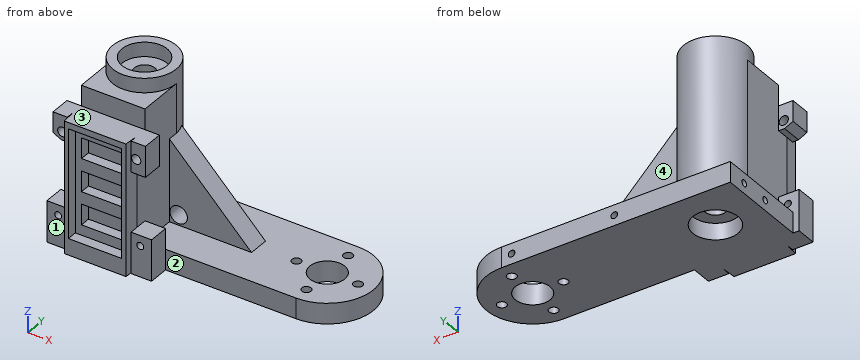
```python
from build123d import *

# Parameters (mm, degrees)
SKETCH1_W                = 26
SKETCH1_H                = 53
SKETCH1_W_2              = 20
SKETCH1_H_2              = 10
BOSS_EXTRUDE1_DEPTH      = 5
SKETCH2_W                = 31
SKETCH2_H                = 59
SKETCH2_W_2              = 26
SKETCH2_H_2              = 53
BOSS_EXTRUDE2_DEPTH      = 10
SKETCH3_W                = 31
SKETCH3_H                = 59
BOSS_EXTRUDE3_DEPTH      = 3
CHAMFER1_SIZE            = 0.5
CHAMFER1_SIZE2           = 7.150333128
SKETCH10_W               = 7
SKETCH10_H               = 15
SKETCH10_R               = 2.25
BOSS_EXTRUDE7_DEPTH      = 10
SKETCH11_W               = 7
SKETCH11_H               = 3
CUT_EXTRUDE4_DEPTH       = 10
CHAMFER2_SIZE            = 2
CHAMFER2_SIZE2           = 4.100607683
BOSS_EXTRUDE8_REACH      = 69.567
SKETCH12_W               = 10
SKETCH12_H               = 15
SKETCH12_R               = 1.676379865
BOSS_EXTRUDE9_START      = -56
SKETCH15_R               = 8.5
SKETCH15_R_2             = 2.25
SKETCH15_R_3             = 11
BOSS_EXTRUDE9_DEPTH      = 5
BOSS_EXTRUDE9_DEPTH_BACK = 5
SKETCH16_R               = 2.25
SKETCH16_R_2             = 8.5
SKETCH16_R_3             = 5
BOSS_EXTRUDE10_DEPTH     = 2
SKETCH17_R               = 5
BOSS_EXTRUDE11_DEPTH     = 64
RIB2_REACH               = 123.175
SKETCH20_WALL_W          = 300.919527638
SKETCH20_WALL_H          = 10
BOSS_EXTRUDE12_DEPTH     = 5
SKETCH22_R               = 15.5
SKETCH22_R_2             = 11
BOSS_EXTRUDE13_DEPTH     = 7
SKETCH23_R               = 4.25
CUT_EXTRUDE5_DEPTH       = 29
SKETCH24_R               = 1.6
CUT_EXTRUDE6_DEPTH       = 8
SKETCH25_R               = 1.6
CUT_EXTRUDE7_DEPTH       = 8


with BuildPart() as part:
    # Sketch1 → Boss-Extrude1 (new body)
    with BuildSketch(Plane(origin=(0, 0, 0), x_dir=(1, 0, 0), z_dir=(0, 1, 0))):
        with Locations((-13, 26.5)):
            Rectangle(SKETCH1_W, SKETCH1_H)
        with Locations((-13, 27)):
            Rectangle(SKETCH1_W_2, SKETCH1_H_2, mode=Mode.SUBTRACT)
        with Locations((-13, 43)):
            Rectangle(SKETCH1_W_2, SKETCH1_H_2, mode=Mode.SUBTRACT)
        with Locations((-13, 11)):
            Rectangle(SKETCH1_W_2, SKETCH1_H_2, mode=Mode.SUBTRACT)
    extrude(amount=BOSS_EXTRUDE1_DEPTH)

    # Sketch2 → Boss-Extrude2 (add)
    with BuildSketch(Plane(origin=(0, 5, 0), x_dir=(1, 0, 0), z_dir=(0, 1, 0))):
        with Locations((-13, 26.5)):
            Rectangle(SKETCH2_W, SKETCH2_H)
        with Locations((-13, 26.5)):
            Rectangle(SKETCH2_W_2, SKETCH2_H_2, mode=Mode.SUBTRACT)
    extrude(amount=-BOSS_EXTRUDE2_DEPTH)

    # Sketch3 → Boss-Extrude3 (add)
    with BuildSketch(Plane(origin=(0, 5, 0), x_dir=(1, 0, 0), z_dir=(0, 1, 0))):
        with Locations((-13, 26.5)):
            Rectangle(SKETCH3_W, SKETCH3_H)
    extrude(amount=BOSS_EXTRUDE3_DEPTH)

    # Chamfer1
    chamfer1_edges = [part.edges().sort_by_distance(p)[0] for p in [
        (-28.5, -5, -26.5),
        (2.5, -5, -26.5),
    ]]
    chamfer1_side = [part.faces().sort_by_distance(p)[0] for p in [
        (-13, -5, -55.333516692),
    ]]
    chamfer(chamfer1_edges, length=CHAMFER1_SIZE, length2=CHAMFER1_SIZE2, reference=chamfer1_side[0])

    # Sketch10 → Boss-Extrude7 (add)
    with BuildSketch(Plane(origin=(0, 8, 0), x_dir=(1, 0, 0), z_dir=(0, 1, 0))):
        with Locations((6, 4.5)):
            Rectangle(SKETCH10_W, SKETCH10_H)
        with Locations(Location((5, 5, 0), (0, 0, 270))):
            Circle(SKETCH10_R, mode=Mode.SUBTRACT)
        with Locations((-32, 4.5)):
            Rectangle(SKETCH10_W, SKETCH10_H)
        with Locations(Location((-31, 5, 0), (0, 0, 90))):
            Circle(SKETCH10_R, mode=Mode.SUBTRACT)
    extrude(amount=-BOSS_EXTRUDE7_DEPTH)

    # Sketch11 → Cut-Extrude4 (cut)
    with BuildSketch(Plane(origin=(0, 8, 0), x_dir=(1, 0, 0), z_dir=(0, 1, 0))):
        with Locations((-32, 10.5)):
            Rectangle(SKETCH11_W, SKETCH11_H)
    extrude(amount=-CUT_EXTRUDE4_DEPTH, mode=Mode.SUBTRACT)

    # Chamfer2
    chamfer2_edges = [part.edges().sort_by_distance(p)[0] for p in [
        (-35.5, 3, -9),
    ]]
    chamfer2_side = [part.faces().sort_by_distance(p)[0] for p in [
        (-35.5, 3, -3),
    ]]
    chamfer(chamfer2_edges, length=CHAMFER2_SIZE, length2=CHAMFER2_SIZE2, reference=chamfer2_side[0])

    # Boss-Extrude8: up to this face of the body (flat: up to its plane)
    boss_extrude8_end = Plane(part.part.faces().sort_by_distance((6, -2, 2.834470546))[0])
    # Sketch12 → Boss-Extrude8 (add, up to the picked face)
    with BuildSketch(Plane(origin=(0, 8, 0), x_dir=(1, 0, 0), z_dir=(0, 1, 0)), mode=Mode.PRIVATE) as boss_extrude8_sk1:
        with Locations((7.5, 48.5)):
            Rectangle(SKETCH12_W, SKETCH12_H)
        with Locations(Location((7, 46, 0), (0, 0, 270))):
            Circle(SKETCH12_R, mode=Mode.SUBTRACT)
    boss_extrude8_tool1 = split(extrude(boss_extrude8_sk1.sketch, amount=-BOSS_EXTRUDE8_REACH, mode=Mode.PRIVATE), bisect_by=boss_extrude8_end, keep=Keep.BOTH, mode=Mode.PRIVATE)
    # Sketch12 → Boss-Extrude8 (add, up to the picked face)
    with BuildSketch(Plane(origin=(0, 8, 0), x_dir=(1, 0, 0), z_dir=(0, 1, 0)), mode=Mode.PRIVATE) as boss_extrude8_sk2:
        with Locations((-33.5, 48.5)):
            Rectangle(SKETCH12_W, SKETCH12_H)
        with Locations(Location((-33, 46, 0), (0, 0, 270))):
            Circle(SKETCH12_R, mode=Mode.SUBTRACT)
    boss_extrude8_tool2 = split(extrude(boss_extrude8_sk2.sketch, amount=-BOSS_EXTRUDE8_REACH, mode=Mode.PRIVATE), bisect_by=boss_extrude8_end, keep=Keep.BOTH, mode=Mode.PRIVATE)
    add(boss_extrude8_tool1.solids().sort_by(Axis((7.531269, 8, -48.656347), (0, -1, 0)))[0])
    add(boss_extrude8_tool2.solids().sort_by(Axis((-33.531269, 8, -48.656347), (0, -1, 0)))[0])

    # Sketch15 → Boss-Extrude9 (add, two sides)
    with BuildSketch(Plane.XY.offset(BOSS_EXTRUDE9_START)) as boss_extrude9_sk:
        with BuildLine():
            Line((-13, 53), (76, 53))
            ThreePointArc((76, 53), (98.5, 30.5), (76, 8))
            Line((76, 8), (-13, 8))
            Line((-13, 8), (-35.5, 8))
            Line((-35.5, 8), (-35.5, 53))
            Line((-35.5, 53), (-13, 53))
        make_face()
        with Locations(Location((76, 30.5, 0), (0, 0, 180))):
            Circle(SKETCH15_R, mode=Mode.SUBTRACT)
        with Locations(Location((76, 45.5, 0), (0, 0, 180))):
            Circle(SKETCH15_R_2, mode=Mode.SUBTRACT)
        with Locations(Location((76, 15.5, 0), (0, 0, 180))):
            Circle(SKETCH15_R_2, mode=Mode.SUBTRACT)
        with Locations(Location((91, 30.5, 0), (0, 0, 180))):
            Circle(SKETCH15_R_2, mode=Mode.SUBTRACT)
        with Locations(Location((61, 30.5, 0), (0, 0, 180))):
            Circle(SKETCH15_R_2, mode=Mode.SUBTRACT)
        with Locations(Location((-13, 30.5, 0), (0, 0, 180))):
            Circle(SKETCH15_R_3, mode=Mode.SUBTRACT)
    extrude(amount=BOSS_EXTRUDE9_DEPTH)
    extrude(boss_extrude9_sk.sketch, amount=-BOSS_EXTRUDE9_DEPTH_BACK)

    # Sketch16 → Boss-Extrude10 (add)
    with BuildSketch(Plane.XY.offset(-51)):
        with BuildLine():
            Line((-35.5, 53), (-35.5, 8))
            Line((-35.5, 8), (12.5, 8))
            Line((12.5, 8), (76, 8))
            ThreePointArc((76, 8), (98.5, 30.5), (76, 53))
            Line((76, 53), (-35.5, 53))
        make_face()
        with Locations(Location((76, 45.5, 0), (0, 0, 180))):
            Circle(SKETCH16_R, mode=Mode.SUBTRACT)
        with Locations(Location((91, 30.5, 0), (0, 0, 180))):
            Circle(SKETCH16_R, mode=Mode.SUBTRACT)
        with Locations(Location((76, 15.5, 0), (0, 0, 180))):
            Circle(SKETCH16_R, mode=Mode.SUBTRACT)
        with Locations(Location((76, 30.5, 0), (0, 0, 180))):
            Circle(SKETCH16_R_2, mode=Mode.SUBTRACT)
        with Locations(Location((61, 30.5, 0), (0, 0, 180))):
            Circle(SKETCH16_R, mode=Mode.SUBTRACT)
        with Locations((-13, 30.5)):
            Circle(SKETCH16_R_3, mode=Mode.SUBTRACT)
    extrude(amount=-BOSS_EXTRUDE10_DEPTH)

    # Sketch17 → Boss-Extrude11 (add)
    with BuildSketch(Plane.XY.offset(-51)):
        with BuildLine():
            Line((-28.5, 30.5), (-28.5, 8))
            Line((-28.5, 8), (2.5, 8))
            Line((2.5, 8), (2.5, 30.5))
            ThreePointArc((2.5, 30.5), (-13, 46), (-28.5, 30.5))
        make_face()
        with Locations((-13, 30.5)):
            Circle(SKETCH17_R, mode=Mode.SUBTRACT)
    extrude(amount=BOSS_EXTRUDE11_DEPTH)

    # Sketch20 wall → Rib2 (add, up to next)
    with BuildSketch(Plane(origin=(22.5, 30.5, -31), x_dir=(-0.707106781187, 0, 0.707106781187), z_dir=(0.707106781187, 0, 0.707106781187)), mode=Mode.PRIVATE) as rib2_sk1:
        Rectangle(SKETCH20_WALL_W, SKETCH20_WALL_H)
    rib2_tool1 = extrude(rib2_sk1.sketch, amount=-RIB2_REACH, mode=Mode.PRIVATE) - part.part
    add(rib2_tool1.solids().sort_by_distance((22.5, 30.5, -31))[0])

    # Sketch21 → Boss-Extrude12 (add)
    with BuildSketch(Plane(origin=(0, 0, -56), x_dir=(-1, 0, 0), z_dir=(0, 0, -1))):
        Polygon((-2, -5), (28, -5), (28.5, 2.150333128), (28.5, -2), (38.5, -2), (38.5, 8), (35.5, 8), (-12.5, 8), (-12.5, -2), (-2.5, -2), (-2.5, 2.150333128), align=None)
    extrude(amount=BOSS_EXTRUDE12_DEPTH)

    # Sketch22 → Boss-Extrude13 (add)
    with BuildSketch(Plane.XY.offset(13)):
        with Locations((-13, 30.5)):
            Circle(SKETCH22_R)
        with Locations((-13, 30.5)):
            Circle(SKETCH22_R_2, mode=Mode.SUBTRACT)
    extrude(amount=BOSS_EXTRUDE13_DEPTH)

    # Sketch23 → Cut-Extrude5 (cut)
    with BuildSketch(Plane(origin=(0, 8, 0), x_dir=(1, 0, 0), z_dir=(0, 1, 0))):
        with Locations(Location((7, 46, 0), (0, 0, 270))):
            Circle(SKETCH23_R)
    extrude(amount=CUT_EXTRUDE5_DEPTH, mode=Mode.SUBTRACT)

    # Sketch24 → Cut-Extrude6 (cut)
    with BuildSketch(Plane.ZY.offset(35.5)):
        with Locations((-56, 28)):
            Circle(SKETCH24_R)
        with Locations((-56, 43)):
            Circle(SKETCH24_R)
    extrude(amount=-CUT_EXTRUDE6_DEPTH, mode=Mode.SUBTRACT)

    # Sketch25 → Cut-Extrude7 (cut)
    with BuildSketch(Plane(origin=(0, 53, 0), x_dir=(1, 0, 0), z_dir=(0, 1, 0))):
        with Locations(Location((71, 56, 0), (0, 0, 270))):
            Circle(SKETCH25_R)
        with Locations(Location((21, 56, 0), (0, 0, 270))):
            Circle(SKETCH25_R)
    extrude(amount=-CUT_EXTRUDE7_DEPTH, mode=Mode.SUBTRACT)


solid = part.part
```
Design review of the part built by this model. Coordinates are the model's own, in mm. Face numbers are marked on the shaded views. A direction names the side the tool comes from. Coordinates: 2 decimals unless noted, no trailing zeros. Order: outer loops, then holes, each group sorted by start corner. A loop starts at its lowest first (then second) coordinate and runs counter-clockwise, first axis right, second up. Notation, with made-up numbers: M 68,55.5 L 98,55.5 A18 ccw 98,85.5 Z; hole C 73.25,52.25 d10. An arc over 180 degrees is marked long. Answer as a JSON object with one key per item and string values. Group by question number.
1) Add section D-D, the plane z = 9.5. Write out the cut boundary in (x, y).
2) Add section B-B, the plane x = 91. Write out the cut boundary in (y, z).
3) Add section A-A, the plane z = -19. Write out the cut boundary in (x, y).
4) For pin 1 (5 mm diameter, centred on x = 33, z = -47.5, fed in from +Y); pin 2 (3 mm diameter, centred on x = -8.5, z = 7, fed in from -Y); pin 3 (1.5 mm diameter, centred on y = 8.5, z = -2, fed in from +X); pin 4 (2.5 mm diameter, centred on x = -33, z = -46, fed in from -Y), all flat-tipped, find the tip position at first contact; note any pin that passes through.
5) Add section C-C, the plane x = 21. Write out the cut boundary in (y, z), then the cut area to 3 significant figures.
6) Tool access review of the marked faces 1, 2, 3 and 4: name each direction out of +Z, -Z, +X, -X, +Y, -Y from which nothing blocks a thin tool from reaching the whole face with its end or side.
7) Wall thickness on L1, parallel to Y at x = 76, z = -55.25; L2, parallel to X at y = 2.75, z = -5; L3, parallel to Y at x = -33, z = -56: over which ranges is each line inside the solid? List them lowest first.
Computed values:
{
 "1": {"outline": "M -28.5,8 L 2.5,8 L 2.5,30.5 A15.5 ccw -28.5,30.5 Z; hole C -13,30.5 d10"},
 "2": {"outline": "M 13.73,-61 L 28.25,-61 L 28.25,-51 L 13.73,-51 Z; M 32.75,-61 L 47.27,-61 L 47.27,-51 L 32.75,-51 Z"},
 "3": {"outline": "M -28.5,2.15 L -28,-5 L -26,-5 L -26,0 L 0,0 L 0,-5 L 2,-5 L 2.5,2.15 L 2.5,25.5 L 10.5,25.5 L 10.5,35.5 L 1.67,35.5 A15.5 ccw -28.5,30.5 Z; hole C -13,30.5 d10"},
 "4": {"pin 1": "stops at y = 35.5", "pin 2": "stops at y = 8", "pin 3": "stops at x = 9.5", "pin 4": "passes through"},
 "5": {"outline": "M 8,-61 L 53,-61 L 53,-57.6 L 45,-57.6 L 45,-54.4 L 53,-54.4 L 53,-51 L 35.5,-51 L 35.5,-29.5 L 25.5,-29.5 L 25.5,-51 L 8,-51 Z", "area": "639 mm^2"},
 "6": {"face 1": "+Z, -Z, -X, -Y", "face 2": "+Z, -Z, +X, -Y", "face 3": "+Z, +X, -X, -Y", "face 4": "+Z, +X, +Y"},
 "7": {"L1": "y = 8 to 13.25, 17.75 to 22, 39 to 43.25, 47.75 to 53", "L2": "x = -35.5 to -33.25, -28.75 to 2.75, 7.25 to 9.5", "L3": "y = -2 to 26.4, 29.6 to 41.4, 44.6 to 53"}
}
